Here's how the part is built. I have some questions about the finished solid (model axes, mm). A direction names the side the tool comes from. Round coordinates to 2 decimals unless told otherwise and drop trailing zeros. Order: outer loops, then holes, each group sorted by start corner. A loop starts at its lowest first (then second) coordinate and runs counter-clockwise, first axis right, second up. Notation, with made-up numbers: M 81.25,55 L 126.25,55 A24 ccw 126.25,69 Z; hole C 3,-21 d1. An arc over 180 degrees is marked long. Write item = value, one per line. Start each with the question number.
Item 1: I want a section at C-C, the plane z = -3.5. List the corners of the cut face in (x, y) for me.
Item 2: I'm going to push flat-ended pins straight in: P1, Ø13.5, axis at x = 42, y = 13, coming from the -Z side; P2, Ø15, axis at y = -6, z = 21, coming from the +X side; P3, Ø6, axis at x = 48.5, y = -23.5, coming from the -Z side. Where does each tip first touch, or does it pass through?
Item 3: Please list where these lines run through material, in increasing order: L1, parallel to X at y = 26.5, z = -0.5; L2, parallel to Y at x = 37.5, z = -4; L3, parallel to Z at x = -12, y = -21.
Item 4: We'd pull the mould along Z, two halves only. Please class faces 5 (the face through (44, -18, 9.522)), 6 (the face through (26, 0, 28.575)), 7 (the face through (-15.12, 0.44, -11.59)): pulls with the +Z half, pulls with the -Z half, needs draft (parallel to the pull), parting line crosses it, or undercut.
Item 5: I want a section at B-B, the plane x = -7. List the corners of the cut face in (y, z) for me.
Item 6: For faces 1 (the face through (60, 0, 9.522)), 2 (the face through (42, -4.762, 0)), 3 (the face through (42, 4.762, 0)), 4 (the face through (19, -31.75, 7)), which set-ups out of +Z, -Z, +X, -X, +Y, -Y let a thin tool reach every point of the face, with its end or its side?
Item 7: I want a section at A-A, the plane y = 9. List the corners of the cut face in (x, z) for me (3 decimals), plus the area to 3 significant figures.
```python
from build123d import *

# Parameters (mm, degrees)
F0_R     = 19.05
F1_DEPTH = 31.75
F2_DEPTH = 4.7625


with BuildPart() as f1:
    # F0 (on Front) → F1 (new body, symmetric)
    with BuildSketch(Plane.XZ):
        with BuildLine():
            ThreePointArc((15.004938, -24.318356), (24.952923, -13.924161), (28.575, 0))
            ThreePointArc((28.575, 0), (31.446927, 6.816322), (38.330852, 9.522202))
            Line((38.330852, 9.522202), (50.8, 9.522202))
            Line((50.8, 9.522202), (50.8, 28.575))
            Line((50.8, 28.575), (0, 28.575))
            ThreePointArc((0, 28.575), (-27.49025, -7.798512), (15.004938, -24.318356))
        make_face()
        Circle(F0_R, mode=Mode.SUBTRACT)
    extrude(amount=F1_DEPTH, both=True)

    # F0 (on Front) → F2 (join, symmetric)
    with BuildSketch(Plane.XZ):
        with BuildLine():
            ThreePointArc((38.330852, 9.522202), (31.446927, 6.816322), (28.575, 0))
            ThreePointArc((28.575, 0), (24.952923, -13.924161), (15.004938, -24.318356))
            Line((15.004938, -24.318356), (69.85, 9.522202))
            Line((69.85, 9.522202), (50.8, 9.522202))
            Line((50.8, 9.522202), (38.330852, 9.522202))
        make_face()
    extrude(amount=F2_DEPTH, both=True)


solid = f1.part
```
Filled in:
q1.outline = M -28.36,-31.75 L -18.73,-31.75 L -18.73,31.75 L -28.36,31.75 Z; M 18.73,-31.75 L 28.36,-31.75 L 28.36,-4.76 L 48.75,-4.76 L 48.75,4.76 L 28.36,4.76 L 28.36,31.75 L 18.73,31.75 Z
q2.P1 = 9.09
q2.P2 = 50.8
q2.P3 = 9.52
q3.L1 = -28.57 to -19.04, 19.04 to 28.57
q3.L2 = -4.76 to 4.76
q3.L3 = -25.93 to -14.8, 14.8 to 25.93
q4.face_5 = pulls with the -Z half
q4.face_6 = pulls with the +Z half
q4.face_7 = undercut
q5.outline = M -31.75,-27.7 L 31.75,-27.7 L 31.75,-17.72 L -31.75,-17.72 Z; M -31.75,17.72 L 31.75,17.72 L 31.75,27.7 L -31.75,27.7 Z
q6.face_1 = +Z, +X, +Y, -Y
q6.face_2 = -Z, +X, -Y
q6.face_3 = -Z, +X, +Y
q6.face_4 = +Z, -Z, +X, -X, -Y
q7.outline = M 0,28.575 A28.575 ccw long 15.005,-24.318 A28.575 ccw 28.575,0 A9.525 cw 38.331,9.522 L 50.8,9.522 L 50.8,28.575 Z; hole C 0,0 d38.1
q7.area = 2,040 mm^2
